Verification items for the finished model (mm, model axes). Give positions to 0.01 mm unless a question says otherwise; leave off trailing zeros. Order: outer loops, then holes, each group sorted by start corner. A loop starts at its lowest first (then second) coordinate and runs counter-clockwise, first axis right, second up. Notation, with made-up numbers: (57.25, 29.5) - (86.25, 29.5) arc R22 cw to (86.25, 43.5) - close; hole circle Ø10 at (-30.75, 62.25). An arc over 180 degrees is marked (long way). Answer as a JSON object with one key per item and string values. Group by question number.
(1) Section check D-D (x = 40.64). Record the boundary of the cut face in (y, z) (1 decimal).
(2) Section check B-B (x = 10.16). Record the boundary of the cut face in (y, z) (1 decimal).
(3) Thickness scan on line 1 (Z direction, x = 29.5, y = 0.55); line 2 (Z direction, x = 11, y = 0.85); line 3 (Z direction, x = 19.5, y = 0.85). Record the ranges inside material, lowest first.
(4) Section check A-A (z = -30.48). Record the boundary of the cut face in (x, y) (1 decimal).
(5) Section check C-C (x = -27.94). Record the boundary of the cut face in (y, z) (1 decimal).
(6) Depth check by flat-ended pin: pin 1 Ø1.6 at (y, z) = (1.5, -47) entering from +X; pin 2 Ø6 at (x, z) = (-43.18, -40.64) entering from +Y (3 decimals). Enter the tip coordinate at first touch or a pass-through.
```python
from build123d import *

# Parameters (mm, degrees)
SKETCH1_R           = 2.15265
SKETCH1_W           = 12.6492
SKETCH1_H           = 3.1242
SKETCH1_R_2         = 2.2225
SKETCH1_R_3         = 1.5875
BOSS_EXTRUDE1_DEPTH = 3.175


with BuildPart() as part:
    # Sketch1 → Boss-Extrude1 (new body)
    with BuildSketch(Plane(origin=(0, 0, 0), x_dir=(1, 0, 0), z_dir=(0, 1, 0))):
        Polygon((63.5, 45.1358), (50.8508, 45.1358), (50.8508, 48.26), (63.5, 48.26), (63.5, 58.42), (-63.5, 58.42), (-63.5, -58.42), (63.5, -58.42), (63.5, -48.26), (50.8508, -48.26), (50.8508, -45.1358), (63.5, -45.1358), align=None)
        with Locations(Location((-50.8, -53.34, 0), (0, 0, 270))):
            Circle(SKETCH1_R, mode=Mode.SUBTRACT)
        with Locations((-44.4246, -46.6979)):
            Rectangle(SKETCH1_W, SKETCH1_H, mode=Mode.SUBTRACT)
        with Locations(Location((-50.8, -40.64, 0), (0, 0, 270))):
            Circle(SKETCH1_R_2, mode=Mode.SUBTRACT)
        with Locations(Location((-43.18, -40.64, 0), (0, 0, 270))):
            Circle(SKETCH1_R_2, mode=Mode.SUBTRACT)
        with Locations(Location((-40.64, -30.48, 0), (0, 0, 270))):
            Circle(SKETCH1_R_3, mode=Mode.SUBTRACT)
        with Locations(Location((-35.56, -40.64, 0), (0, 0, 270))):
            Circle(SKETCH1_R_2, mode=Mode.SUBTRACT)
        with Locations(Location((-27.94, -40.64, 0), (0, 0, 270))):
            Circle(SKETCH1_R_2, mode=Mode.SUBTRACT)
        with Locations((-19.0246, -46.6979)):
            Rectangle(SKETCH1_W, SKETCH1_H, mode=Mode.SUBTRACT)
        with Locations(Location((-20.32, -40.64, 0), (0, 0, 270))):
            Circle(SKETCH1_R_2, mode=Mode.SUBTRACT)
        with Locations(Location((-12.7, -40.64, 0), (0, 0, 270))):
            Circle(SKETCH1_R_2, mode=Mode.SUBTRACT)
        with Locations(Location((-5.08, -40.64, 0), (0, 0, 270))):
            Circle(SKETCH1_R_2, mode=Mode.SUBTRACT)
        with Locations((6.3754, -46.6979)):
            Rectangle(SKETCH1_W, SKETCH1_H, mode=Mode.SUBTRACT)
        with Locations(Location((2.54, -40.64, 0), (0, 0, 270))):
            Circle(SKETCH1_R_2, mode=Mode.SUBTRACT)
        with Locations(Location((10.16, -40.64, 0), (0, 0, 270))):
            Circle(SKETCH1_R_2, mode=Mode.SUBTRACT)
        with Locations(Location((17.78, -40.64, 0), (0, 0, 270))):
            Circle(SKETCH1_R_2, mode=Mode.SUBTRACT)
        with Locations(Location((25.4, -40.64, 0), (0, 0, 270))):
            Circle(SKETCH1_R_2, mode=Mode.SUBTRACT)
        with Locations((31.7754, -46.6979)):
            Rectangle(SKETCH1_W, SKETCH1_H, mode=Mode.SUBTRACT)
        with Locations(Location((50.8, -53.34, 0), (0, 0, 270))):
            Circle(SKETCH1_R, mode=Mode.SUBTRACT)
        with Locations(Location((33.02, -40.64, 0), (0, 0, 270))):
            Circle(SKETCH1_R_2, mode=Mode.SUBTRACT)
        with Locations(Location((40.64, -40.64, 0), (0, 0, 270))):
            Circle(SKETCH1_R_2, mode=Mode.SUBTRACT)
        with Locations(Location((40.64, -30.48, 0), (0, 0, 270))):
            Circle(SKETCH1_R_3, mode=Mode.SUBTRACT)
        with Locations(Location((-40.64, 30.48, 0), (0, 0, 270))):
            Circle(SKETCH1_R_3, mode=Mode.SUBTRACT)
        with Locations(Location((-50.8, 40.64, 0), (0, 0, 270))):
            Circle(SKETCH1_R_2, mode=Mode.SUBTRACT)
        with Locations(Location((-43.18, 40.64, 0), (0, 0, 270))):
            Circle(SKETCH1_R_2, mode=Mode.SUBTRACT)
        with Locations(Location((-35.56, 40.64, 0), (0, 0, 270))):
            Circle(SKETCH1_R_2, mode=Mode.SUBTRACT)
        with Locations(Location((-27.94, 40.64, 0), (0, 0, 270))):
            Circle(SKETCH1_R_2, mode=Mode.SUBTRACT)
        with Locations((-44.4246, 46.6979)):
            Rectangle(SKETCH1_W, SKETCH1_H, mode=Mode.SUBTRACT)
        with Locations(Location((-50.8, 53.34, 0), (0, 0, 270))):
            Circle(SKETCH1_R, mode=Mode.SUBTRACT)
        with Locations(Location((-20.32, 40.64, 0), (0, 0, 270))):
            Circle(SKETCH1_R_2, mode=Mode.SUBTRACT)
        with Locations(Location((-12.7, 40.64, 0), (0, 0, 270))):
            Circle(SKETCH1_R_2, mode=Mode.SUBTRACT)
        with Locations(Location((-5.08, 40.64, 0), (0, 0, 270))):
            Circle(SKETCH1_R_2, mode=Mode.SUBTRACT)
        with Locations((-19.0246, 46.6979)):
            Rectangle(SKETCH1_W, SKETCH1_H, mode=Mode.SUBTRACT)
        with Locations(Location((2.54, 40.64, 0), (0, 0, 270))):
            Circle(SKETCH1_R_2, mode=Mode.SUBTRACT)
        with Locations(Location((10.16, 40.64, 0), (0, 0, 270))):
            Circle(SKETCH1_R_2, mode=Mode.SUBTRACT)
        with Locations(Location((17.78, 40.64, 0), (0, 0, 270))):
            Circle(SKETCH1_R_2, mode=Mode.SUBTRACT)
        with Locations(Location((25.4, 40.64, 0), (0, 0, 270))):
            Circle(SKETCH1_R_2, mode=Mode.SUBTRACT)
        with Locations((6.3754, 46.6979)):
            Rectangle(SKETCH1_W, SKETCH1_H, mode=Mode.SUBTRACT)
        with Locations(Location((33.02, 40.64, 0), (0, 0, 270))):
            Circle(SKETCH1_R_2, mode=Mode.SUBTRACT)
        with Locations(Location((40.64, 30.48, 0), (0, 0, 270))):
            Circle(SKETCH1_R_3, mode=Mode.SUBTRACT)
        with Locations(Location((40.64, 40.64, 0), (0, 0, 270))):
            Circle(SKETCH1_R_2, mode=Mode.SUBTRACT)
        with Locations((31.7754, 46.6979)):
            Rectangle(SKETCH1_W, SKETCH1_H, mode=Mode.SUBTRACT)
        with Locations(Location((50.8, 53.34, 0), (0, 0, 270))):
            Circle(SKETCH1_R, mode=Mode.SUBTRACT)
    extrude(amount=BOSS_EXTRUDE1_DEPTH)


solid = part.part
```
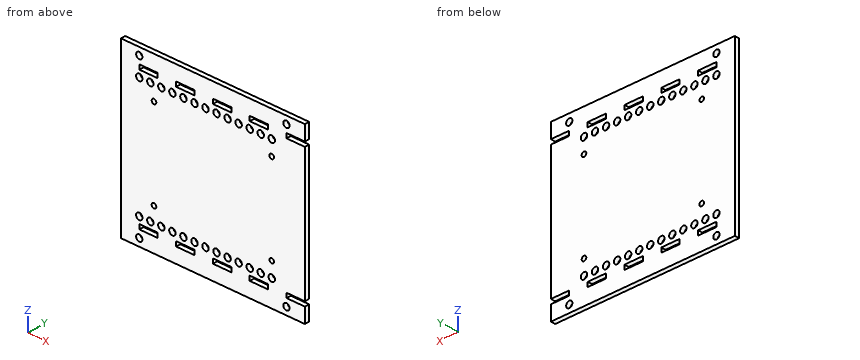
Solutions:
{
 "1": {"outline": "(0, -58.4) - (3.2, -58.4) - (3.2, -42.9) - (0, -42.9) - close; (0, -38.4) - (3.2, -38.4) - (3.2, -32.1) - (0, -32.1) - close; (0, -28.9) - (3.2, -28.9) - (3.2, 28.9) - (0, 28.9) - close; (0, 32.1) - (3.2, 32.1) - (3.2, 38.4) - (0, 38.4) - close; (0, 42.9) - (3.2, 42.9) - (3.2, 58.4) - (0, 58.4) - close"},
 "2": {"outline": "(0, -58.4) - (3.2, -58.4) - (3.2, -48.3) - (0, -48.3) - close; (0, -45.1) - (3.2, -45.1) - (3.2, -42.9) - (0, -42.9) - close; (0, -38.4) - (3.2, -38.4) - (3.2, 38.4) - (0, 38.4) - close; (0, 42.9) - (3.2, 42.9) - (3.2, 45.1) - (0, 45.1) - close; (0, 48.3) - (3.2, 48.3) - (3.2, 58.4) - (0, 58.4) - close"},
 "3": {"line 1": "z = -58.42 to -48.26, -45.14 to 45.14, 48.26 to 58.42", "line 2": "z = -58.42 to -48.26, -45.14 to -42.7, -38.58 to 38.58, 42.7 to 45.14, 48.26 to 58.42", "line 3": "z = -58.42 to -42.05, -39.23 to 39.23, 42.05 to 58.42"},
 "4": {"outline": "(-63.5, 0) - (-42.2, 0) - (-42.2, 3.2) - (-63.5, 3.2) - close; (-39.1, 0) - (39.1, 0) - (39.1, 3.2) - (-39.1, 3.2) - close; (42.2, 0) - (63.5, 0) - (63.5, 3.2) - (42.2, 3.2) - close"},
 "5": {"outline": "(0, -58.4) - (3.2, -58.4) - (3.2, -42.9) - (0, -42.9) - close; (0, -38.4) - (3.2, -38.4) - (3.2, 38.4) - (0, 38.4) - close; (0, 42.9) - (3.2, 42.9) - (3.2, 58.4) - (0, 58.4) - close"},
 "6": {"pin 1": "stops at x = 50.85", "pin 2": "stops at y = 3.175"}
}
